```python
from build123d import *

# Parameters (mm, degrees)
F1_DEPTH = 25.4
F2_W     = 71.67115435
F2_H     = 9.5259128138
F3_DEPTH = 25.4
F4_DEPTH = 90.678
F5_W     = 2.7504333318
F5_H     = 2.2891710663
F5_H_2   = 10.414
F5_W_2   = 28.4633595034
F5_H_3   = 2.5368289337
F5_W_3   = 1.8062071648
F5_H_4   = 2.5342966719
F6_DEPTH = 254


with BuildPart() as f1:
    # F0 (on Top) → F1 (new body)
    with BuildSketch(Plane.XY):
        Polygon((13.3816469461, 0), (-10.2063324302, 0), (-26.9900802523, -33.3406925201), (29.2581655085, -33.3406925201), align=None)
    extrude(amount=F1_DEPTH)

    # F2 (on face) → F3 (cut)
    with BuildSketch(Plane(origin=(0, 0, 0), x_dir=(-1, 0, 0), z_dir=(0, 1, 0))):
        with Locations((-2.7216915041, 13.6072267778)):
            Rectangle(F2_W, F2_H)
    extrude(amount=-F3_DEPTH, mode=Mode.SUBTRACT)

    # F4 (add): a face of the model
    f4_faces = [f1.faces().sort_by_distance(p)[0] for p in [
        (1.1340426281, -33.3406925201, 12.7),
    ]]
    extrude(f4_faces, amount=F4_DEPTH)

    # F5 (on face) → F6 (cut)
    with BuildSketch(Plane.XZ.offset(124.0186925201)):
        with Locations((16.251562838, 6.0353870775)):
            Rectangle(F5_W, F5_H)
        with Locations((16.251562838, 12.3869726107)):
            Rectangle(F5_W, F5_H_2)
        with Locations((0.6446664204, 12.3869726107)):
            Rectangle(F5_W_2, F5_H_2)
        with Locations((16.251562838, 18.8623870775)):
            Rectangle(F5_W, F5_H_3)
        with Locations((-14.4901169138, 5.9128242747)):
            Rectangle(F5_W_3, F5_H_4)
        with Locations((-14.4901169138, 12.3869726107)):
            Rectangle(F5_W_3, F5_H_2)
        with Locations((-14.4901169138, 18.8623870775)):
            Rectangle(F5_W_3, F5_H_3)
    extrude(amount=-F6_DEPTH, mode=Mode.SUBTRACT)


solid = f1.part
```
Model file for the job. Use its own axes, mm. A direction names the side the tool comes from. Coordinates: 2 decimals unless noted, no trailing zeros. Order: outer loops, then holes, each group sorted by start corner. A loop starts at its lowest first (then second) coordinate and runs counter-clockwise, first axis right, second up. Notation, with made-up numbers: (88.5, 14) -> (142.5, 14) arc R32 ccw to (142.5, 45) -> close; hole circle Ø5 at (14.25, 13.5). An arc over 180 degrees is marked (long way). Answer as a JSON object with one key per item and string values. Group by question number.
1) Drill centre lines: L1, parallel to X at y = -81, z = 5.75; L2, parallel to Z at x = -3, y = -84; L3, parallel to Z at x = 15, y = -79. Where is each one in solid material? Low to high.
2) Pull direction X, two halves, no side cores. Call faces 4 (the face through (2, 0, 4)), 5 (the face through (-26.99, -78, 13)), 6 (the face through (16, -64, 20.131)): +X half, -X half, draft (parallel to the pull), parting line (faces both ways), or undercut.
3) Which spindle directions (+Z, -Z, +X, -X, +Y, -Y) get a long thin tool onto all of the face, cutting with end or side? Do faces 1 (the face through (16, -64, 4.891)), 2 (the face through (22, -25.4, 14)), 3 (the face through (1, -61, 25.4)). Say none if no direction does.
4) Cut at A-A, the plane y = -83.5. Write the cut outline in (x, z), then the cut area to 3 significant figures.
5) Cut at D-D, the plane z = 23.5. Write the cut outline in (x, y).
6) Cut at B-B, the plane z = 15.5. Write the cut outline in (x, y), then the cut area to 3 significant figures.
7) Cut at C-C, the plane x = 6.5. Write the cut outline in (y, z), then the cut area to 3 significant figures.
8) Flat gauge pins, fed straight in: pin 1 (6.5 mm diameter, centred on x = 22, z = 14.5, fed in from +Y); pin 2 (4 mm diameter, centred on y = -27, z = 3.5, fed in from -X) (3 decimals). Where does each tip first touch, or does it go through?
Check values:
{
 "1": {"L1": "x = -26.99 to -15.39, -13.59 to 14.88, 17.63 to 29.26", "L2": "z = 0 to 7.18, 17.59 to 25.4", "L3": "z = 0 to 4.89, 20.13 to 25.4"},
 "2": {"face 4": "draft", "face 5": "-X half", "face 6": "undercut"},
 "3": {"face 1": "+Y, -Y", "face 2": "+X, -X, +Y", "face 3": "+Z, +X, -X, +Y, -Y"},
 "4": {"outline": "(-26.99, 0) -> (29.26, 0) -> (29.26, 25.4) -> (-26.99, 25.4) -> close; hole (-15.39, 4.65) -> (-13.59, 4.65) -> (-13.59, 7.18) -> (14.88, 7.18) -> (14.88, 4.89) -> (17.63, 4.89) -> (17.63, 20.13) -> (14.88, 20.13) -> (14.88, 17.59) -> (-13.59, 17.59) -> (-13.59, 20.13) -> (-15.39, 20.13) -> close", "area": "1,060 mm²"},
 "5": {"outline": "(-26.99, -124.02) -> (29.26, -124.02) -> (29.26, -33.34) -> (13.38, 0) -> (-10.21, 0) -> (-26.99, -33.34) -> close"},
 "6": {"outline": "(-26.99, -124.02) -> (-15.39, -124.02) -> (-15.39, -25.4) -> (-22.99, -25.4) -> (-26.99, -33.34) -> close; (17.63, -124.02) -> (29.26, -124.02) -> (29.26, -33.34) -> (25.48, -25.4) -> (17.63, -25.4) -> close", "area": "2,260 mm²"},
 "7": {"outline": "(-124.02, 0) -> (0, 0) -> (0, 7.18) -> (-124.02, 7.18) -> close; (-124.02, 17.59) -> (-25.4, 17.59) -> (-25.4, 18.37) -> (0, 18.37) -> (0, 25.4) -> (-124.02, 25.4) -> close", "area": "1,840 mm²"},
 "8": {"pin 1": "stops at y = -25.4", "pin 2": "stops at x = -24.805"}
}
